Verification items for the finished model (mm, model axes). Face numbers are marked on the shaded views. Coordinates: 2 decimals unless noted, no trailing zeros. Order: outer loops, then holes, each group sorted by start corner. A loop starts at its lowest first (then second) coordinate and runs counter-clockwise, first axis right, second up. Notation, with made-up numbers: (15.25, 75.25) -> (53.25, 75.25) arc R25 cw to (53.25, 106.25) -> close; hole circle Ø11 at (-16.5, 11). An arc over 180 degrees is marked (long way). Write item = value, one per line. Start each with the question number.
1. Release check for a two-part mould opening along Z. For the marked faces 1, 2, 3 and 4 record: +Z half, -Z half, draft (parallel to the pull), parting line (faces both ways), or undercut.
2. Go/stop test with flat-tipped pins: P1, Ø2, axis at x = 1.5, z = 12, coming from the -Y side; P2, Ø4, axis at x = 1, z = 0, coming from the +Y side; P3, Ø3, axis at x = 0, z = -20, coming from the +Y side. Record where each tip stops, or that it passes through.
3. Cross-section at D-D on z = 0. Record the cut outline in (x, y).
4. Cross-section at C-C on y = 2.25. Record the cut outline in (x, z).
5. Cross-section at A-A on z = -20. Record the cut outline in (x, y).
6. Thickness scan on line 1 along Z through (x, y) = (-0.25, 9.5); line 2 along X through (y, z) = (23.75, 0); line 3 along X through (y, z) = (1.75, -20). Record the ranges inside material, lowest first. Write a range as from..to.
7. Cross-section at B-B on x = 0. Record the cut outline in (y, z).
from build123d import *

# Parameters (mm, degrees)
SKETCH_2_W      = 19
SKETCH_2_H      = 62
SKETCH_2_R      = 1.7
EXTRUDE_1_DEPTH = 4
SKETCH_3_R      = 7.15
SKETCH_3_R_2    = 4.15
EXTRUDE_2_DEPTH = 25
FILLET_1_R      = 3
FILLET_2_R      = 1


with BuildPart() as part:
    # 草图2 → 凸台-拉伸1 (new body)
    with BuildSketch(Plane(origin=(0, 0, 0), x_dir=(1, 0, 0), z_dir=(0, 1, 0))):
        Rectangle(SKETCH_2_W, SKETCH_2_H)
        with Locations(Location((0, 20, 0), (0, 0, 270))):
            Circle(SKETCH_2_R, mode=Mode.SUBTRACT)
        with Locations(Location((0, -20, 0), (0, 0, 270))):
            Circle(SKETCH_2_R, mode=Mode.SUBTRACT)
    extrude(amount=EXTRUDE_1_DEPTH)

    # 草图3 → 凸台-拉伸2 (add)
    with BuildSketch(Plane(origin=(0, 4, 0), x_dir=(1, 0, 0), z_dir=(0, 1, 0))):
        with Locations(Location((0, 0, 0), (0, 0, 270))):
            Circle(SKETCH_3_R)
        with Locations(Location((0, 0, 0), (0, 0, 270))):
            Circle(SKETCH_3_R_2, mode=Mode.SUBTRACT)
    extrude(amount=EXTRUDE_2_DEPTH)

    # 圆角1
    fillet_1_edges = [part.edges().sort_by_distance(p)[0] for p in [
        (-9.5, 2, -31),
        (9.5, 2, -31),
        (9.5, 2, 31),
        (-9.5, 2, 31),
    ]]
    fillet(fillet_1_edges, radius=FILLET_1_R)

    # 圆角2
    fillet_2_edges = [part.edges().sort_by_distance(p)[0] for p in [
        (0, 29, -7.15),
        (0, 4, -7.15),
    ]]
    fillet(fillet_2_edges, radius=FILLET_2_R)


solid = part.part
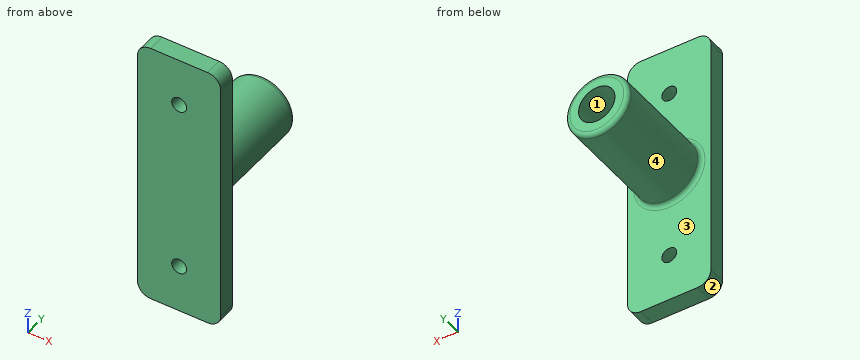
Worked out:
q1.face_1 = undercut
q1.face_2 = -Z half
q1.face_3 = draft
q1.face_4 = parting line
q2.P1 = 0
q2.P2 = 4
q2.P3 = through
q3.outline = (-9.5, 0) -> (9.5, 0) -> (9.5, 4) -> (8.15, 4) arc R1 cw to (7.15, 5) -> (7.15, 28) arc R1 ccw to (6.15, 29) -> (4.15, 29) -> (4.15, 4) -> (-4.15, 4) -> (-4.15, 29) -> (-6.15, 29) arc R1 ccw to (-7.15, 28) -> (-7.15, 5) arc R1 cw to (-8.15, 4) -> (-9.5, 4) -> close
q4.outline = (-9.5, -28) arc R3 ccw to (-6.5, -31) -> (6.5, -31) arc R3 ccw to (9.5, -28) -> (9.5, 28) arc R3 ccw to (6.5, 31) -> (-6.5, 31) arc R3 ccw to (-9.5, 28) -> close; hole circle Ø3.4 at (0, -20); hole circle Ø3.4 at (0, 20)
q5.outline = (-9.5, 0) -> (-1.7, 0) -> (-1.7, 4) -> (-9.5, 4) -> close; (1.7, 0) -> (9.5, 0) -> (9.5, 4) -> (1.7, 4) -> close
q6.line_1 = -7.15..-4.14, 4.14..7.15
q6.line_2 = -7.15..-4.15, 4.15..7.15
q6.line_3 = -9.5..-1.7, 1.7..9.5
q7.outline = (0, -31) -> (4, -31) -> (4, -21.7) -> (0, -21.7) -> close; (0, -18.3) -> (4, -18.3) -> (4, -8.15) arc R1 cw to (5, -7.15) -> (28, -7.15) arc R1 ccw to (29, -6.15) -> (29, -4.15) -> (4, -4.15) -> (4, 4.15) -> (29, 4.15) -> (29, 6.15) arc R1 ccw to (28, 7.15) -> (5, 7.15) arc R1 cw to (4, 8.15) -> (4, 18.3) -> (0, 18.3) -> close; (0, 21.7) -> (4, 21.7) -> (4, 31) -> (0, 31) -> close
